Can you work these out from the model? Positions are in its coordinate system, mm. A direction names the side the tool comes from. Coordinates: 2 decimals unless noted, no trailing zeros. Order: outer loops, then holes, each group sorted by start corner. A loop starts at its lowest first (then second) coordinate and runs counter-clockwise, first axis right, second up. Notation, with made-up numbers: (-26.75, 67.25) -> (7.25, 67.25) arc R38 ccw to (7.25, 106.25) -> close; hole circle Ø1 at (64, 85). An arc over 180 degrees is marked (long way). Write item = value, one per line.
```python
from build123d import *

# Parameters (mm, degrees)
EXTRUDE_1_DEPTH         = 16
HOLE_WIZARD_4_2_4_2_1_D = 4.2
FILLET_1_R              = 0.5


with BuildPart() as part:
    # Эскиз1 → Бобышка-Вытянуть1 (new body)
    with BuildSketch(Plane.XY.offset(8)):
        with BuildLine():
            Line((-9.756337345, 8.497441256), (-12.271369771, 6.893092394))
            ThreePointArc((-12.271369771, 6.893092394), (-13.850276142, 2.692375438), (-10.26, 0))
            Line((-10.26, 0), (0, 0))
            Line((0, 0), (0, 2))
            Line((0, 2), (-10.26, 2))
            ThreePointArc((-10.26, 2), (-11.930342376, 3.252602477), (-11.195770963, 5.206946729))
            Line((-11.195770963, 5.206946729), (-8.680738537, 6.81129559))
            ThreePointArc((-8.680738537, 6.81129559), (-8.718896971, 7.97309132), (-9.756337345, 8.497441256))
        make_face()
    extrude(amount=-EXTRUDE_1_DEPTH)

    # Диаметр отверстия Ø4.2 (4.2)1 (through all)
    with Locations(Plane(origin=(0, 2, 0), x_dir=(1, 0, 0), z_dir=(0, 1, 0))):
        with Locations((-4, 4), (-4, -4)):
            Hole(HOLE_WIZARD_4_2_4_2_1_D / 2)

    # Скругление1
    fillet_1_edges = [part.edges().sort_by_distance(p)[0] for p in [
        (0, 2, 0),
        (0, 0, 0),
    ]]
    fillet(fillet_1_edges, radius=FILLET_1_R)


solid = part.part
```
Item 1: I want a section at A-A, the plane x = -4. Please give me the cut outline in (y, z).
A:
outline = (0, -8) -> (2, -8) -> (2, -6.1) -> (0, -6.1) -> close; (0, -1.9) -> (2, -1.9) -> (2, 1.9) -> (0, 1.9) -> close; (0, 6.1) -> (2, 6.1) -> (2, 8) -> (0, 8) -> close
Item 2: If we mould it in two halves opening along Z, with no side actions, what happens to faces 3 (the cylindrical face through (-5.94, 0.99, -3.2)), 4 (the cylindrical face through (-8.71, 7.96, 0.11)), 5 (the cylindrical face through (-4.969, 0.986, 5.863)), 6 (the flat face through (-9, 1, 8))? For each: pulls with the +Z half, pulls with the -Z half, needs draft (parallel to the pull), parting line crosses it, or undercut.
A:
face_3 = undercut
face_4 = needs draft
face_5 = undercut
face_6 = pulls with the +Z half
Item 3: For faces 1 (the flat face through (-5, 0, 0)), 2 (the flat face through (-5, 2, 0)), which set-ups out of +Z, -Z, +X, -X, +Y, -Y let a thin tool reach every point of the face, with its end or its side?
A:
face_1 = +Z, -Z, +X, -X, -Y
face_2 = +Z, -Z, +X
Item 4: I want a section at B-B, the plane z = 4. Please give me the cut outline in (x, y).
A:
outline = (-12.27, 6.89) arc R3.74 ccw to (-10.26, 0) -> (-6.1, 0) -> (-6.1, 2) -> (-10.26, 2) arc R1.74 cw to (-11.2, 5.21) -> (-8.68, 6.81) arc R1.14 ccw to (-9.76, 8.5) -> close; (-1.9, 0) -> (-0.5, 0) arc R0.5 ccw to (0, 0.5) -> (0, 1.5) arc R0.5 ccw to (-0.5, 2) -> (-1.9, 2) -> close
Item 5: I want a section at D-D, the plane y = 5. Please give me the cut outline in (x, z), plus the area to 3 significant figures.
A:
outline = (-13.78, -8) -> (-11.46, -8) -> (-11.46, 8) -> (-13.78, 8) -> close
area = 37.1 mm2
Item 6: If I drill on probe 1 along Z at (x, y) = (-4, 1.5); probe 2 along Y at (x, z) = (-5.5, 6.75); probe 3 along Y at (x, z) = (-11.5, -0.75), over which ranges is the centre line in solid material (lowest first)?
A:
probe_1 = -8 to -6.1, -1.9 to 1.9, 6.1 to 8
probe_2 = 0 to 2
probe_3 = 0.21 to 2.52, 4.96 to 7.39
Item 7: I want a section at C-C, the plane z = 1.25. Please give me the cut outline in (x, y), plus the area to 3 significant figures.
A:
outline = (-12.27, 6.89) arc R3.74 ccw to (-10.26, 0) -> (-0.5, 0) arc R0.5 ccw to (0, 0.5) -> (0, 1.5) arc R0.5 ccw to (-0.5, 2) -> (-10.26, 2) arc R1.74 cw to (-11.2, 5.21) -> (-8.68, 6.81) arc R1.14 ccw to (-9.76, 8.5) -> close
area = 41.3 mm2
Item 8: I'm going to push flat-ended pins straight in: P1, Ø2, axis at y = 6.5, z = -6.5, coming from the -X side; P2, Ø1, axis at y = 3, z = 3.5, coming from the +X side; P3, Ø3, axis at x = -7.5, z = -3, coming from the +Y side (3 decimals). Where does each tip first touch, or does it pass through?
A:
P1 = -13.56
P2 = -11.48
P3 = 8.275
